Study the drawing (mm; zero at the part's minimum x, y, z) and answer. Round coordinates to 2 decimals unless told otherwise and drop trailing zeros. Order: outer loops, then holes, each group sorted by start corner. A loop starts at its lowest first (then second) coordinate and runs counter-clockwise, first axis right, second up. Notation, with made-up numbers: (-32.75, 83) - (-13.75, 83) arc R11 ccw to (-13.75, 90) - close; hole circle Ø8 at (-8, 47.5). An arc over 180 degrees is marked (long way). Put each result on its own line as item: value. Start each with the question number.
Q1. Section B-B on x = 5.1 is taken. Give the vertices of the cut face in (y, z) (3 decimals).
Q2. This flat-tipped pin is pushed along its axis until it touches: pin 1 Ø4.5 at (x, y) = (184.9, 123.5) entering from +Z. Where does it stop, or does it pass through?
Q3. Section A-A on y = 123.5 is taken. Give the vertices of the cut face in (x, z) (3 decimals), then the cut area to 3 significant figures.
Q4. Find the intervals of material crossed by line 1 along Y through (x, z) = (5.1, 1.2) (3 decimals); line 2 along X through (y, z) = (122.5, 2), in increasing order. Write a range as from..to.
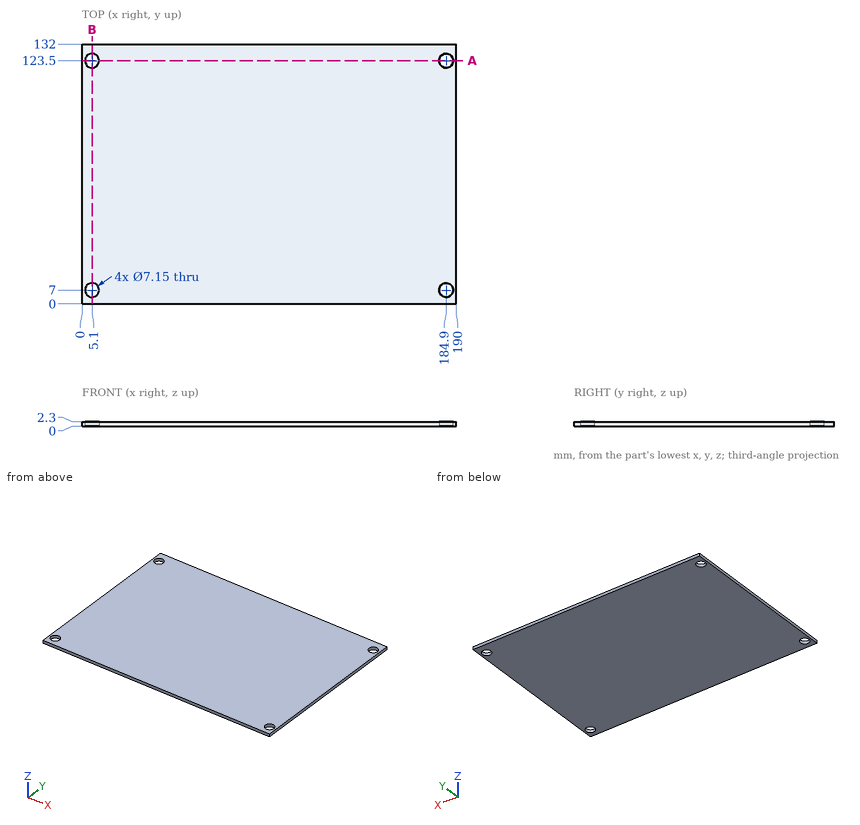
Findings:
1. outline: (0, 0) - (3.425, 0) - (3.425, 2.3) - (0, 2.3) - close; (10.575, 0) - (119.925, 0) - (119.925, 2.3) - (10.575, 2.3) - close; (127.075, 0) - (132, 0) - (132, 2.3) - (127.075, 2.3) - close
2. pin 1: through
3. outline: (0, 0) - (1.525, 0) - (1.525, 2.3) - (0, 2.3) - close; (8.675, 0) - (181.325, 0) - (181.325, 2.3) - (8.675, 2.3) - close; (188.475, 0) - (190, 0) - (190, 2.3) - (188.475, 2.3) - close
3. area: 404 mm2
4. line 1: 0..3.425, 10.575..119.925, 127.075..132
4. line 2: 0..1.67, 8.53..181.47, 188.33..190
